Source: CAD feature listing. Evaluate the final solid. Frame: model axes, mm. A direction names the side the tool comes from. Round coordinates to 2 decimals unless told otherwise and drop trailing zeros. Order: outer loops, then holes, each group sorted by start corner. A loop starts at its lowest first (then second) coordinate and runs counter-clockwise, first axis right, second up. Notation, with made-up numbers: M 60,72 L 114,72 A22 ccw 114,94 Z; hole C 10,-7 d6. An arc over 180 degrees is marked long. Use one line per item in the form item = value. Start each with the question number.
Q1. Section A-A (y = 0). Return the cut outline in (x, z).
Q2. Reachability of faces 1 (the flat face through (13.169, -4.793, 19.72)), 2 (the cylindrical face through (3.69, -7.1, 44.93)), 3 (the flat face through (-13.143, -4.783, 19.72)) from +Z, -Z, +X, -X, +Y, -Y: full face, straight path, thin tool, end or side. Return the list, or none.
Q3. Material intervals for probe 1 along X at (y, z) = (9.5, 10.5); probe 2 along Z at (x, y) = (-2, 14); probe 3 along Z at (x, y) = (0, -5.85), sorted ascending.
Q4. Section D-D (x = 5). Return the cut outline in (y, z) (3 decimals).
Q5. Pull-direction query (X, two-part tool) for faces 4 (the cylindrical face through (1.636, -5.794, 44.785)), 5 (the cylindrical face through (0, -15, 20)), 6 (the cylindrical face through (13.009, 7.468, 19.72)), 7 (the flat face through (-2.43, -13.77, 19.72)); classes: pulls with the +X half, pulls with the -X half, needs draft (parallel to the pull), parting line crosses it, or undercut.
Q6. Section B-B (x = 0). Return the cut outline in (y, z), plus the area to 3 significant figures.
Q7. Section C-C (z = 27.5). Return the cut outline in (x, y).
Q8. Contact query for flat-ended pins moving along their axis: pin 1 (1.5 mm diameter, centred on y = -6.5, z = 7.5, fed in from -X); pin 2 (2 mm diameter, centred on x = 4.5, z = 12.5, fed in from +Y); pin 3 (12 mm diameter, centred on x = -7, z = 6.5, fed in from +Y); pin 4 (6.5 mm diameter, centred on x = 0, y = 0, fed in from +Z). Output: stop coordinate, or through.
from build123d import *

# Parameters (mm, degrees)
ESQUISSE1_R             = 60
BOSS_EXTRU_1_DEPTH      = 40
CUT_EXTRUDE4_DEPTH      = 94.808315196
CIRPATTERN1_COUNT       = 10
SKETCH4_R               = 8
BOSS_EXTRUDE1_DEPTH     = 10
SKETCH5_R               = 4
CUT_EXTRUDE5_DEPTH      = 99.488578018
CUT_EXTRUDE6_START      = -20
CUT_EXTRUDE6_DEPTH      = 20
CIRPATTERN2_COUNT       = 15
CUT_EXTRUDE7_DEPTH      = 20
CIRPATTERN3_COUNT       = 15
CUT_EXTRUDE8_DEPTH      = 94.808315196
CUT_EXTRUDE8_DEPTH_BACK = 94.808315196
SKETCH8_OUTSIDE_W       = 157.384
SKETCH8_OUTSIDE_H       = 157.384
CUT_EXTRUDE9_REACH      = 56.071
CUT_EXTRUDE9_END_RADIUS = 8
SKETCH9_R               = 1.65


with BuildPart() as part:
    # Esquisse1 → Boss.-Extru.1 (new body)
    with BuildSketch(Plane.XY):
        Circle(ESQUISSE1_R)
    extrude(amount=BOSS_EXTRU_1_DEPTH)

    # Sketch3 → Cut-Extrude4 (cut, symmetric)
    with BuildSketch(Plane.XY):
        with BuildLine():
            Line((-3.943348831, 23.180571367), (-7.5, 44.087980221))
            ThreePointArc((-7.5, 44.087980221), (-6.481937987, 48.04148707), (-2.856459957, 49.918339681))
            ThreePointArc((-2.856459957, 49.918339681), (0, 50), (2.856459957, 49.918339681))
            ThreePointArc((2.856459957, 49.918339681), (6.481937987, 48.04148707), (7.5, 44.087980221))
            Line((7.5, 44.087980221), (3.943348831, 23.180571367))
            ThreePointArc((3.943348831, 23.180571367), (0, 19.85139176), (-3.943348831, 23.180571367))
        make_face()
    cut_extrude4 = extrude(amount=CUT_EXTRUDE4_DEPTH, both=True, mode=Mode.SUBTRACT)

    # CirPattern1: Cut-Extrude4 ×10 about axis
    cirpattern1_axis = Axis((0, 0, 0), (0, 0, 1))
    for i in range(1, CIRPATTERN1_COUNT):
        add(cut_extrude4.rotate(cirpattern1_axis, i * 360 / CIRPATTERN1_COUNT), mode=Mode.SUBTRACT)

    # Sketch4 → Boss-Extrude1 (add)
    with BuildSketch(Plane.XY.offset(40)):
        Circle(SKETCH4_R)
    extrude(amount=BOSS_EXTRUDE1_DEPTH)

    # Sketch5 → Cut-Extrude5 (cut, through all)
    with BuildSketch(Plane.XY.offset(50)):
        Circle(SKETCH5_R)
    extrude(amount=-CUT_EXTRUDE5_DEPTH, mode=Mode.SUBTRACT)

    # Sketch6 → Cut-Extrude6 (cut)
    with BuildSketch(Plane.XY.offset(40).offset(CUT_EXTRUDE6_START)):
        with BuildLine():
            Line((14.752685571, 55.057772098), (15.529142706, 57.955549577))
            ThreePointArc((15.529142706, 57.955549577), (12.986376836, 58.577760427), (10.41889066, 59.088465181))
            Line((10.41889066, 59.088465181), (9.897946127, 56.134041922))
            ThreePointArc((9.897946127, 56.134041922), (12.337057994, 55.648872406), (14.752685571, 55.057772098))
        make_face()
    cut_extrude6 = extrude(amount=CUT_EXTRUDE6_DEPTH, mode=Mode.SUBTRACT)

    # CirPattern2: Cut-Extrude6 ×15 about axis
    cirpattern2_axis = Axis((0, 0, 0), (0, 0, 1))
    for i in range(1, CIRPATTERN2_COUNT):
        add(cut_extrude6.rotate(cirpattern2_axis, i * 360 / CIRPATTERN2_COUNT), mode=Mode.SUBTRACT)

    # Sketch7 → Cut-Extrude7 (cut)
    with BuildSketch(Plane(origin=(0, 0, 0), x_dir=(-1, 0, 0), z_dir=(0, 0, -1))):
        with BuildLine():
            Line((-2.617163242, 59.942893295), (-2.48630508, 56.94574863))
            ThreePointArc((-2.48630508, 56.94574863), (0, 57), (2.48630508, 56.94574863))
            Line((2.48630508, 56.94574863), (2.617163242, 59.942893295))
            ThreePointArc((2.617163242, 59.942893295), (0, 60), (-2.617163242, 59.942893295))
        make_face()
    cut_extrude7 = extrude(amount=-CUT_EXTRUDE7_DEPTH, mode=Mode.SUBTRACT)

    # CirPattern3: Cut-Extrude7 ×15 about axis
    cirpattern3_axis = Axis((0, 0, 0), (0, 0, 1))
    for i in range(1, CIRPATTERN3_COUNT):
        add(cut_extrude7.rotate(cirpattern3_axis, i * 360 / CIRPATTERN3_COUNT), mode=Mode.SUBTRACT)

    # Sketch8 outside → Cut-Extrude8 (cut, two sides: drawn at the far end of the back side and taken through both)
    with BuildSketch(Plane.XY.offset(40).offset(-CUT_EXTRUDE8_DEPTH_BACK)):
        Rectangle(SKETCH8_OUTSIDE_W, SKETCH8_OUTSIDE_H)
        with BuildLine():
            Line((-2.604722665, 14.772116295), (-2.25742631, 12.802500789))
            ThreePointArc((-2.25742631, 12.802500789), (-6.5, 11.258330249), (-9.958577761, 8.356238926))
            Line((-9.958577761, 8.356238926), (-11.490666647, 9.641814145))
            ThreePointArc((-11.490666647, 9.641814145), (-12.990381057, 7.5), (-14.095389312, 5.13030215))
            Line((-14.095389312, 5.13030215), (-12.21600407, 4.446261863))
            ThreePointArc((-12.21600407, 4.446261863), (-13, 0), (-12.21600407, -4.446261863))
            Line((-12.21600407, -4.446261863), (-14.095389312, -5.13030215))
            ThreePointArc((-14.095389312, -5.13030215), (-12.990381057, -7.5), (-11.490666647, -9.641814145))
            Line((-11.490666647, -9.641814145), (-9.958577761, -8.356238926))
            ThreePointArc((-9.958577761, -8.356238926), (-6.5, -11.258330249), (-2.25742631, -12.802500789))
            Line((-2.25742631, -12.802500789), (-2.604722665, -14.772116295))
            ThreePointArc((-2.604722665, -14.772116295), (0, -15), (2.604722665, -14.772116295))
            Line((2.604722665, -14.772116295), (2.25742631, -12.802500789))
            ThreePointArc((2.25742631, -12.802500789), (6.5, -11.258330249), (9.958577761, -8.356238926))
            Line((9.958577761, -8.356238926), (11.490666647, -9.641814145))
            ThreePointArc((11.490666647, -9.641814145), (12.990381057, -7.5), (14.095389312, -5.13030215))
            Line((14.095389312, -5.13030215), (12.21600407, -4.446261863))
            ThreePointArc((12.21600407, -4.446261863), (13, 0), (12.21600407, 4.446261863))
            Line((12.21600407, 4.446261863), (14.095389312, 5.13030215))
            ThreePointArc((14.095389312, 5.13030215), (12.990381057, 7.5), (11.490666647, 9.641814145))
            Line((11.490666647, 9.641814145), (9.958577761, 8.356238926))
            ThreePointArc((9.958577761, 8.356238926), (6.5, 11.258330249), (2.25742631, 12.802500789))
            Line((2.25742631, 12.802500789), (2.604722665, 14.772116295))
            ThreePointArc((2.604722665, 14.772116295), (0, 15), (-2.604722665, 14.772116295))
        make_face(mode=Mode.SUBTRACT)
    extrude(amount=CUT_EXTRUDE8_DEPTH + CUT_EXTRUDE8_DEPTH_BACK, mode=Mode.SUBTRACT)

    # Cut-Extrude9: up to this cylinder (the profile starts inside it)
    cut_extrude9_end = Plane(origin=(0, 0, 45), z_dir=(0, 0, -1)) * Cylinder(CUT_EXTRUDE9_END_RADIUS, 129.142, mode=Mode.PRIVATE)
    # Sketch9 → Cut-Extrude9 (cut, up to the surface)
    with BuildSketch(Plane(origin=(0, 0, 0), x_dir=(1, 0, 0), z_dir=(0, 1, 0)), mode=Mode.PRIVATE) as cut_extrude9_sk1:
        with Locations(Location((0, -45, 0), (0, 0, 270))):
            Circle(SKETCH9_R)
    cut_extrude9_tool1 = extrude(cut_extrude9_sk1.sketch, amount=-CUT_EXTRUDE9_REACH, mode=Mode.PRIVATE) & cut_extrude9_end
    add(cut_extrude9_tool1.solids().sort_by_distance((0, 0, 45))[0], mode=Mode.SUBTRACT)


solid = part.part
Results list:
q1.outline = M -13,0 L -4,0 L -4,50 L -8,50 L -8,40 L -13,40 Z; M 4,0 L 13,0 L 13,40 L 8,40 L 8,50 L 4,50 Z
q2.face_1 = +Z, -Z, +X
q2.face_2 = +Z
q2.face_3 = +Z, -Z, -X
q3.probe_1 = -11.61 to -11.32, -8.87 to 8.87, 11.32 to 11.61
q3.probe_2 = 0 to 40
q3.probe_3 = 0 to 43.35, 46.65 to 50
q4.outline = M -12,0 L 12,0 L 12,40 L 6.245,40 L 6.245,50 L -6.245,50 L -6.245,40 L -12,40 Z
q5.face_4 = undercut
q5.face_5 = parting line crosses it
q5.face_6 = pulls with the +X half
q5.face_7 = pulls with the -X half
q6.outline = M -15,0 L -4,0 L -4,43.35 L -8,43.35 L -8,40 L -15,40 Z; M -8,46.65 L -4,46.65 L -4,50 L -8,50 Z; M 4,0 L 15,0 L 15,40 L 8,40 L 8,50 L 4,50 Z
q6.area = 947 mm2
q7.outline = M -14.1,-5.13 A15 ccw -11.49,-9.64 L -9.96,-8.36 A13 ccw -2.26,-12.8 L -2.6,-14.77 A15 ccw 2.6,-14.77 L 2.26,-12.8 A13 ccw 9.96,-8.36 L 11.49,-9.64 A15 ccw 14.1,-5.13 L 12.22,-4.45 A13 ccw 12.22,4.45 L 14.1,5.13 A15 ccw 11.49,9.64 L 9.96,8.36 A13 ccw 2.26,12.8 L 2.6,14.77 A15 ccw -2.6,14.77 L -2.26,12.8 A13 ccw -9.96,8.36 L -11.49,9.64 A15 ccw -14.1,5.13 L -12.22,4.45 A13 ccw -12.22,-4.45 Z; hole C 0,0 d8
q8.pin_1 = -13.85
q8.pin_2 = 12.52
q8.pin_3 = 14.97
q8.pin_4 = through
